Source: CAD feature listing. Evaluate the final solid. Frame: model axes, mm. A direction names the side the tool comes from. Give positions to 0.01 mm unless a question says otherwise; leave off trailing zeros. Write each loop counter-clockwise with the first axis right and the second up, starting at its lowest first coordinate (ties: lowest second). Pieces come first, ordered by that corner, then holes. Notation, with made-up numbers: (-31, -14) -> (16, -14) arc R16 ccw to (16, -3) -> close; hole circle Ø4 at (68.25, -18). An arc over 180 degrees is marked (long way). Answer as a JSON object with one key per item and string values. Group by question number.
Item 1: Pull-direction query (Z, two-part tool) for faces 5 (the face through (5, 29, -22)), 6 (the face through (0.6, 31, -23)), 7 (the face through (0, 14, -20.25)), 8 (the face through (4.512, 28.768, 26.446)); classes: pulls with the +Z half, pulls with the -Z half, needs draft (parallel to the pull), parting line crosses it, or undercut.
Item 2: First-contact query: pin 1 Ø1 at (x, y) = (5.5, 20) entering from +Z; pin 2 Ø1 at (x, y) = (4.5, 25.5) entering from -Z; pin 3 Ø7 at (x, z) = (4, 24) entering from +Y; pin 4 Ø1.5 at (x, z) = (7, 2) entering from -Y. Flat tips, straight axial feed; report the tip coordinate or a pass-through.
Item 3: Ray query, probe 1 along X at (y, z) = (28, -24); probe 2 along Z at (x, y) = (5, 28.2); probe 3 along X at (y, z) = (34, 10). Return the intervals inside material, ascending. Write a range as from..to.
Item 4: Section query D-D on x = 8.5. Return the cut outline in (y, z), plus the area to 3 significant figures.
Item 5: Section query B-B on z = -24.25. Return the cut outline in (x, y), plus the area to 3 significant figures.
Item 6: Section query A-A on z = 24.25. Return the cut outline in (x, y).
Item 7: Section query C-C on y = 4. Return the cut outline in (x, z).
Item 8: Access query for faces 1 (the face through (-0.6, 31, 24)), 2 (the face through (-0.6, 31, -23)), 3 (the face through (0, 32, 24)), 4 (the face through (3.75, 5, 23)). Directions: +Z, -Z, +X, -X, +Y, -Y. A direction counts if a zero-diameter tool reaches every point of the face in a straight line with its end or side. Return the directions, or none.
Autodesk Inventor part; units mm, degrees
ref_plane "YZ Plane" through (0, 0, 0) normal (1, 0, 0) x (0, 1, 0)
ref_plane "XZ Plane" through (0, 0, 0) normal (0, 1, 0) x (-1, 0, 0)
ref_plane "XY Plane" through (0, 0, 0) normal (0, 0, 1) x (1, 0, 0)
sketch "Sketch1" plane through (0, 0, 0) normal (0, 1, 0) x (-1, 0, 0)
  line L0 (-10, 20.25) -> (10, 20.25)
  line L1 (10, 20.25) -> (10, -20.25)
  line L2 (10, -20.25) -> (-10, -20.25)
  line L3 (-10, -20.25) -> (-10, 20.25)
  point P0 (0, 0)
  point P1 (0, 20.25)
  point P2 (10, 0)
  dimension "s_width" = 40.5
  dimension "s_depth" = 20
extrude "Extrusion1" add sketch "Sketch1" along normal blind 38
sketch "Sketch2" plane through (-10, 0, 20.25) normal (0, 0, 1) x (1, 0, 0)
  line L0 (0, 38) -> (20, 38) construction
  line L1 (10, 38) -> (10, 0) construction
  line L2 (0, 27.5) -> (20, 27.5)
  line L3 (20, 27.5) -> (20, 30)
  line L4 (20, 30) -> (0, 30)
  line L5 (0, 30) -> (0, 27.5)
  dimension "s_land_thickness" = 2.5
  dimension "s_land_dist_top" = 8
extrude "Extrusion2" add sketch "Sketch2" along normal blind 6.5 and the other way blind 47
sketch "Sketch3" plane through (-10, 30, 20.25) normal (0, 1, 0) x (1, 0, 0)
  line L0 (0, -6.5) -> (0, 0) construction
  line L1 (20, 0) -> (20, -6.5) construction
  circle A0 centre (5, -4) radius 2.25
  line L2 (0, -4) -> (20, -4) construction
  line L3 (20, -6.5) -> (0, -6.5)
  line L4 (0, 47) -> (0, 40.5) construction
  line L5 (0, 44.5) -> (20, 44.5) construction
  line L6 (20, 47) -> (20, 40.5) construction
  line L7 (0, 47) -> (20, 47)
  circle A1 centre (15, 44.5) radius 2.25
  circle A2 centre (15, -4) radius 2.25
  circle A3 centre (5, 44.5) radius 2.25
  point P0 (10, 20.25)
  dimension "s_hole_dia" = 4.5
  dimension "s_hole_front_dist" = 2.5
  dimension "d13" = 2.5
  dimension "s_hole_side_dist" = 2.75
  dimension "d42" = 2.75
extrude "Extrusion3" cut sketch "Sketch3" against normal up to next
sketch "Sketch4" plane through (-10, 0, 20.25) normal (0, 0, 1) x (1, 0, 0)
  line L0 (6.25, 3) -> (13.75, 3)
  line L1 (13.75, 3) -> (13.75, 8)
  line L2 (13.75, 8) -> (6.25, 8)
  line L3 (6.25, 8) -> (6.25, 3)
  line L4 (10, 0) -> (10, 27.5) construction
  line L5 (20, 27.5) -> (0, 27.5) construction
  line L6 (20, 0) -> (0, 0) construction
  point P0 (10, 8)
  dimension "s_cable_height" = 5
  dimension "s_cable_width" = 7.5
  dimension "s_cable_dist_bottom" = 3
extrude "Extrusion4" add sketch "Sketch4" along normal blind 6.5
sketch "Sketch5" plane through (-10, 38, 20.25) normal (0, 0, 1) x (1, 0, 0)
  line L0 (0, 0) -> (20, 0) construction
  line L1 (10, 0) -> (10, -8) construction
  line L2 (0, -8) -> (20, -8) construction
  line L3 (0, -8) -> (0, 0) construction
  line L4 (0, -4) -> (20, -4) construction
  line L5 (20, -8) -> (20, 0) construction
  line L6 (9.4, -8) -> (10.6, -8)
  line L7 (10.6, -8) -> (10.6, -6)
  line L8 (10.6, -6) -> (9.4, -6)
  line L9 (9.4, -6) -> (9.4, -8)
  line L10 (20, -8) -> (0, -8)
  point P0 (10, -38)
  dimension "s_land_pin_thickness" = 2
  dimension "d27" = 1.2
extrude "Extrusion5" add sketch "Sketch5" against normal up to surface (53.5 mm away) from surface at 6.5
sketch "Sketch6" plane through (0, 38, 0) normal (0, 1, 0) x (1, 0, 0)
  circle A0 centre (0, -10.25) radius 4.5
  line L0 (0, 0) -> (0, -26.75) construction
  line L1 (-10, -26.75) -> (10, -26.75) construction
  line L2 (10, 20.25) -> (-10, 20.25)
  line L3 (-10, -20.25) -> (10, -20.25)
  dimension "s_shaft_dia" = 9
  dimension "s_shaft_front_dist" = 10
extrude "Extrusion6" add sketch "Sketch6" along normal blind 4
sketch "Sketch8" plane through (0, 42, 10.25) normal (0, 1, 0) x (1, 0, 0)
  circle A0 centre (0, 0) radius 2.5
  circle A1 centre (0, 0) radius 4.5 construction
  point P0 (0, 10.25)
  dimension "d39" = 5
extrude "Extrusion8" cut sketch "Sketch8" against normal blind 12
equation "\"s_width\" = servo_width"
equation "\"s_depth\" = servo_depth"
equation "\"s_height\" = servo_height"
equation "\"s_land_dist_top\" = servo_mount_dist_top"
equation "\"s_land\" = servo_mount_length"
equation "\"d7\" = s_land + s_width"
equation "\"s_hole_dia\" = servo_mount_hole_diameter"
equation "\"s_hole_front_dist\" = servo_mount_hole_front_distance"
equation "\"d13\" = s_hole_front_dist"
equation "\"s_hole_side_dist\" = servo_mount_hole_side_distance"
equation "\"d42\" = s_hole_side_dist"
equation "\"s_cable_height\" = servo_cable_heigth"
equation "\"s_cable_width\" = servo_cable_width"
equation "\"s_cable_dist_bottom\" = servo_cable_distance_bottom"
equation "\"d24\" = servo_cable_length"
equation "\"s_land_pin_thickness\" = servo_mount_pin_height"
equation "\"d27\" = servo_mount_pin_thickness"
equation "\"s_shaft_front_dist\" = servo_shaft_front_distance"
equation "\"s_shaft_height\" = servo_shaft_height"
equation "\"servo_depth\" = 20"
equation "\"servo_height\" = 38"
equation "\"servo_width\" = 40.5"
equation "\"servo_mount_length\" = 6.5"
equation "\"servo_mount_hole_diameter\" = 4.5"
equation "\"servo_mount_hole_front_distance\" = 2.5"
equation "\"servo_mount_hole_side_distance\" = 2.75"
equation "\"servo_mount_pin_thickness\" = 1.2"
equation "\"servo_mount_pin_height\" = 2"
equation "\"servo_shaft_height\" = 4"
equation "\"servo_mount_dist_top\" = 8"
equation "\"servo_shaft_front_distance\" = 10"
equation "\"servo_cable_width\" = 7.5"
equation "\"servo_cable_length\" = 6.5"
equation "\"servo_cable_distance_bottom\" = 3"
equation "\"servo_cable_heigth\" = 5"
properties part number "Servo"
Worked answers:
{
 "1": {"face 5": "undercut", "face 6": "needs draft", "face 7": "pulls with the -Z half", "face 8": "undercut"},
 "2": {"pin 1": "z = 20.25", "pin 2": "z = -20.25", "pin 3": "y = 32", "pin 4": "y = 0"},
 "3": {"probe 1": "-10..-7.24, -2.76..2.76, 7.24..10", "probe 2": "-26.75..-26.5, -22..22, 26.5..26.75", "probe 3": "-10..-2.49, 2.49..10"},
 "4": {"outline": "(0, -20.25) -> (27.5, -20.25) -> (27.5, -26.75) -> (30, -26.75) -> (30, -20.25) -> (38, -20.25) -> (38, 20.25) -> (30, 20.25) -> (30, 26.75) -> (27.5, 26.75) -> (27.5, 20.25) -> (0, 20.25) -> close", "area": "1,570 mm^2"},
 "5": {"outline": "(-10, 27.5) -> (-7.25, 27.5) -> (-7.25, 30) -> (-10, 30) -> close; (-2.75, 27.5) -> (2.75, 27.5) -> (2.75, 30) -> (0.6, 30) -> (0.6, 32) -> (-0.6, 32) -> (-0.6, 30) -> (-2.75, 30) -> close; (7.25, 27.5) -> (10, 27.5) -> (10, 30) -> (7.25, 30) -> close", "area": "29.9 mm^2"},
 "6": {"outline": "(-10, 27.5) -> (-7.25, 27.5) -> (-7.25, 30) -> (-10, 30) -> close; (-3.75, 3) -> (3.75, 3) -> (3.75, 8) -> (-3.75, 8) -> close; (-2.75, 27.5) -> (2.75, 27.5) -> (2.75, 30) -> (0.6, 30) -> (0.6, 32) -> (-0.6, 32) -> (-0.6, 30) -> (-2.75, 30) -> close; (7.25, 27.5) -> (10, 27.5) -> (10, 30) -> (7.25, 30) -> close"},
 "7": {"outline": "(-10, -20.25) -> (10, -20.25) -> (10, 20.25) -> (3.75, 20.25) -> (3.75, 26.75) -> (-3.75, 26.75) -> (-3.75, 20.25) -> (-10, 20.25) -> close"},
 "8": {"face 1": "+Z, -X, +Y", "face 2": "-Z, -X, +Y", "face 3": "+Z, +X, -X, +Y", "face 4": "+Z, +X, -Y"}
}
